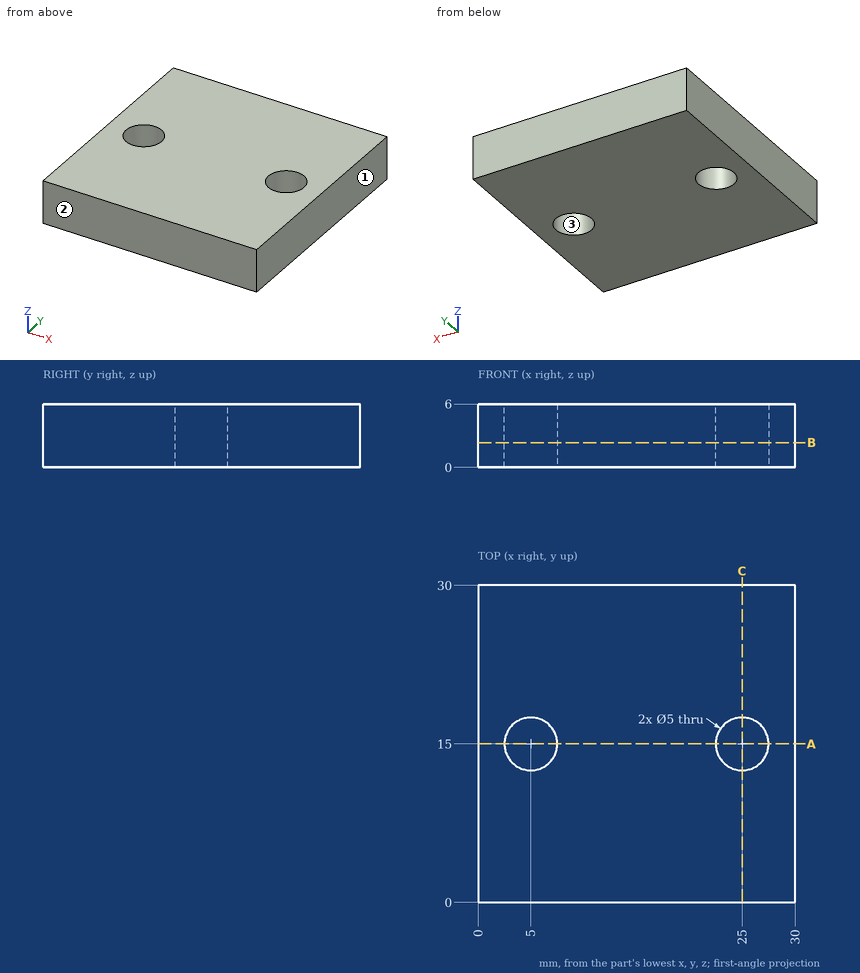
Could you check a few things on this drawing? It's one solid part, dimensions in mm from its lowest x, y, z. Give positions to 0.01 mm unless a question says otherwise; leave off trailing zeros. Write each loop counter-clockwise with the first axis right and the second up, starting at its lowest first coordinate (ties: lowest second). Pieces come first, ordered by that corner, then holes. Notation, with made-up numbers: (37.5, 70) -> (54.5, 70) arc R8 cw to (54.5, 82) -> close; hole circle Ø2 at (66.25, 35). An arc over 180 degrees is marked (long way). Answer as CSV lines item,"result". Start each with the question number.
(1) If we section it at C-C, the plane x = 25: Write out the boundary of the cut face in (y, z).
(2) If we section it at A-A, the plane y = 15: Write out the boundary of the cut face in (x, z), and give its area (3 significant figures).
(3) I'm going to push flat-ended pins straight in: pin 1 Ø6.5 at (x, y) = (25, 15) entering from -Z; pin 2 Ø3 at (x, y) = (5, 15) entering from +Z. Where does each tip first touch, or does it pass through?
(4) If we mould it in two halves opening along X, with no side actions, what happens to the marked faces 1, 2 and 3? For each: +X half, -X half, draft (parallel to the pull), parting line (faces both ways), or undercut.
(5) If we section it at B-B, the plane z = 2.35: Write out the boundary of the cut face in (x, y), and give its area (3 significant figures).
(6) Please list where these lines run through material, in increasing order: line 1 (Y direction, x = 25, z = 3.2); line 2 (X direction, y = 15.75, z = 3.25); line 3 (X direction, y = 16, z = 2.05).
Answer list:
1,outline,"(0, 0) -> (12.5, 0) -> (12.5, 6) -> (0, 6) -> close; (17.5, 0) -> (30, 0) -> (30, 6) -> (17.5, 6) -> close"
2,outline,"(0, 0) -> (2.5, 0) -> (2.5, 6) -> (0, 6) -> close; (7.5, 0) -> (22.5, 0) -> (22.5, 6) -> (7.5, 6) -> close; (27.5, 0) -> (30, 0) -> (30, 6) -> (27.5, 6) -> close"
2,area,"120 mm^2"
3,pin 1,"z = 0"
3,pin 2,"through"
4,face 1,"+X half"
4,face 2,"draft"
4,face 3,"undercut"
5,outline,"(0, 0) -> (30, 0) -> (30, 30) -> (0, 30) -> close; hole circle Ø5 at (5, 15); hole circle Ø5 at (25, 15)"
5,area,"861 mm^2"
6,line 1,"0 to 12.5, 17.5 to 30"
6,line 2,"0 to 2.62, 7.38 to 22.62, 27.38 to 30"
6,line 3,"0 to 2.71, 7.29 to 22.71, 27.29 to 30"
